```python
from build123d import *

# Parameters (mm, degrees)
SKETCH_31_W              = 54.5
SKETCH_31_H              = 38
EXTRUDE_11_DEPTH         = 4
SKETCH_32_W              = 4
SKETCH_32_H              = 38
EXTRUDE_12_DEPTH         = 28.5
SKETCH_33_W              = 16
SKETCH_33_H              = 38
EXTRUDE_13_DEPTH         = 4
SKETCH_34_W              = 15
SKETCH_34_H              = 4
EXTRUDE_14_DEPTH         = 28.5
HOLE_WIZARD_M2_5_1_D     = 2.9
HOLE_WIZARD_M2_5_1_DEPTH = 10
HOLE_WIZARD_M2_5_1_TIP   = 0.871247898
HOLE_WIZARD_M2_5_2_D     = 2.9
HOLE_WIZARD_M2_5_2_DEPTH = 10
HOLE_WIZARD_M2_5_2_TIP   = 0.871247898
HOLE_WIZARD_M2_5_3_D     = 2.9
HOLE_WIZARD_M2_5_3_DEPTH = 10
HOLE_WIZARD_M2_5_3_TIP   = 0.871247898
HOLE_WIZARD_M4_1_D       = 4.5
HOLE_WIZARD_M4_1_DEPTH   = 10
HOLE_WIZARD_M4_1_TIP     = 1.351936393
SKETCH_46_W              = 43
SKETCH_46_H              = 32.5
CUT_EXTRUDE_4_DEPTH      = 4


with BuildPart() as part:
    # 스케치31 → 보스-돌출11 (new body)
    with BuildSketch(Plane(origin=(0, 0, 0), x_dir=(1, 0, 0), z_dir=(0, 1, 0))):
        Rectangle(SKETCH_31_W, SKETCH_31_H)
    extrude(amount=EXTRUDE_11_DEPTH)

    # 스케치32 → 보스-돌출12 (add)
    with BuildSketch(Plane.XZ):
        with Locations((25.25, 0)):
            Rectangle(SKETCH_32_W, SKETCH_32_H)
        with Locations((-25.25, 0)):
            Rectangle(SKETCH_32_W, SKETCH_32_H)
    extrude(amount=EXTRUDE_12_DEPTH)

    # 스케치33 → 보스-돌출13 (add)
    with BuildSketch(Plane.XZ.offset(28.5)):
        with Locations((-35.25, 0)):
            Rectangle(SKETCH_33_W, SKETCH_33_H)
        with Locations((35.25, 0)):
            Rectangle(SKETCH_33_W, SKETCH_33_H)
    extrude(amount=-EXTRUDE_13_DEPTH)

    # 스케치34 → 보스-돌출14 (add)
    with BuildSketch(Plane.XZ):
        with Locations((-15.75, 17)):
            Rectangle(SKETCH_34_W, SKETCH_34_H)
    extrude(amount=EXTRUDE_14_DEPTH)

    # M2.5 여유 구멍1
    with Locations(Plane(origin=(0, 4, 0), x_dir=(1, 0, 0), z_dir=(0, 1, 0))):
        with Locations((8, 8), (8, -4), (-16, -4), (-16, 8)):
            Hole(HOLE_WIZARD_M2_5_1_D / 2, depth=HOLE_WIZARD_M2_5_1_DEPTH)
            with Locations((0, 0, -(HOLE_WIZARD_M2_5_1_DEPTH + HOLE_WIZARD_M2_5_1_TIP / 2))):  # 118° drill point
                Cone(0, HOLE_WIZARD_M2_5_1_D / 2, HOLE_WIZARD_M2_5_1_TIP, mode=Mode.SUBTRACT)

    # M2.5 여유 구멍2
    with Locations(Plane(origin=(27.25, 0, 0), x_dir=(0, 0, -1), z_dir=(1, 0, 0))):
        with Locations((-4, -6.25)):
            Hole(HOLE_WIZARD_M2_5_2_D / 2, depth=HOLE_WIZARD_M2_5_2_DEPTH)
            with Locations((0, 0, -(HOLE_WIZARD_M2_5_2_DEPTH + HOLE_WIZARD_M2_5_2_TIP / 2))):  # 118° drill point
                Cone(0, HOLE_WIZARD_M2_5_2_D / 2, HOLE_WIZARD_M2_5_2_TIP, mode=Mode.SUBTRACT)

    # M2.5 여유 구멍3
    with Locations(Plane.ZY.offset(27.25)):
        with Locations((4, -6.25), (-8, -6.25)):
            Hole(HOLE_WIZARD_M2_5_3_D / 2, depth=HOLE_WIZARD_M2_5_3_DEPTH)
            with Locations((0, 0, -(HOLE_WIZARD_M2_5_3_DEPTH + HOLE_WIZARD_M2_5_3_TIP / 2))):  # 118° drill point
                Cone(0, HOLE_WIZARD_M2_5_3_D / 2, HOLE_WIZARD_M2_5_3_TIP, mode=Mode.SUBTRACT)

    # M4 여유 구멍1
    with Locations(Plane(origin=(0, -24.5, 0), x_dir=(1, 0, 0), z_dir=(0, 1, 0))):
        with Locations((36.25, 10), (36.25, -10), (-36.25, -10), (-36.25, 10)):
            Hole(HOLE_WIZARD_M4_1_D / 2, depth=HOLE_WIZARD_M4_1_DEPTH)
            with Locations((0, 0, -(HOLE_WIZARD_M4_1_DEPTH + HOLE_WIZARD_M4_1_TIP / 2))):  # 118° drill point
                Cone(0, HOLE_WIZARD_M4_1_D / 2, HOLE_WIZARD_M4_1_TIP, mode=Mode.SUBTRACT)

    # 스케치46 → 컷-돌출4 (cut)
    with BuildSketch(Plane.XY.offset(19)):
        with Locations((21.75, -12.25)):
            Rectangle(SKETCH_46_W, SKETCH_46_H)
    extrude(amount=-CUT_EXTRUDE_4_DEPTH, mode=Mode.SUBTRACT)


solid = part.part
```
Part model, mm, in its own coordinate system. A direction names the side the tool comes from. Give positions to 0.01 mm unless a question says otherwise; leave off trailing zeros. Write each loop counter-clockwise with the first axis right and the second up, starting at its lowest first coordinate (ties: lowest second). Pieces come first, ordered by that corner, then holes. Notation, with made-up numbers: M 21,11 L 53,11 A16 ccw 53,34 Z; hole C 74,2.25 d1. An arc over 180 degrees is marked long. Use CSV: the item, a comma, the result in double quotes.
Item 1: Pull direction Z, two halves, no side cores. Call faces 1 (the face through (35.04, -26.528, 8.103)), 2 (the face through (23.25, -14, -2)), 3 (the face through (25, -10, 15)): +Z half, -Z half, draft (parallel to the pull), parting line (faces both ways), or undercut.
Taken from the geometry:
face 1,"undercut"
face 2,"draft"
face 3,"+Z half"
Item 2: Drill centre lines: probe 1 along X at (y, z) = (2.2, -8); probe 2 along Z at (x, y) = (-16, 1); probe 3 along X at (y, z) = (-26, 10). Where is each one in solid material? Low to high.
Taken from the geometry:
probe 1,"x = -27.25 to -17.45, -14.55 to 6.55, 9.45 to 27.25"
probe 2,"z = -19 to -9.45, -6.55 to 2.55, 5.45 to 19"
probe 3,"x = -43.25 to -38.5, -34 to -23.25, 23.25 to 34, 38.5 to 43.25"
Item 3: Slice it at D-D on y = -4. Write the cut outline in (x, z), plus the area to 3 significant figures.
Taken from the geometry:
outline,"M -27.25,-19 L -23.25,-19 L -23.25,15 L -8.25,15 L -8.25,19 L -27.25,19 Z; M 23.25,-19 L 27.25,-19 L 27.25,15 L 23.25,15 Z"
area,"348 mm²"
Item 4: Which spindle directions (+Z, -Z, +X, -X, +Y, -Y) get a long thin tool onto all of the face, cutting with end or side? Do faces 4 (the face through (-25.22, -6.19, -6.55)), 5 (the face through (-8.25, -14, 17)), 6 (the face through (27.25, -10, -2)), 7 (the face through (-23.25, -14, -2)). Say none if no direction does.
Taken from the geometry:
face 4,"-X"
face 5,"+Z, -Z, +X, -Y"
face 6,"+Z, -Z, +X, +Y"
face 7,"-Z, -Y"
Item 5: Slice it at B-B on x = -16. Write the cut outline in (y, z), plus the area to 3 significant figures.
Taken from the geometry:
outline,"M -28.5,15 L 0,15 L 0,5.45 L 4,5.45 L 4,19 L -28.5,19 Z; M 0,-19 L 4,-19 L 4,-9.45 L 0,-9.45 Z; M 0,-6.55 L 4,-6.55 L 4,2.55 L 0,2.55 Z"
area,"243 mm²"
Item 6: Pin check, flat tips, straight feed: P1, Ø3.5, axis at y = -6.25, z = -8, coming from the +X side; P2, Ø1.7, axis at y = -6.25, z = 4, coming from the -X side; P3, Ø10, axis at x = 22, y = -19.5, coming from the +Z side; P4, Ø1.5, axis at y = -3, z = 13, coming from the -X side. Stop position of each tip, or through.
Taken from the geometry:
P1,"stops at x = 27.25"
P2,"passes through"
P3,"stops at z = 15"
P4,"stops at x = -27.25"
Item 7: Slice it at C-C on z = 10. Write the cut outline in (x, y).
Taken from the geometry:
outline,"M -43.25,-28.5 L -38.5,-28.5 L -38.5,-24.5 L -43.25,-24.5 Z; M -34,-28.5 L -23.25,-28.5 L -23.25,0 L 23.25,0 L 23.25,-28.5 L 34,-28.5 L 34,-24.5 L 27.25,-24.5 L 27.25,4 L -27.25,4 L -27.25,-24.5 L -34,-24.5 Z; M 38.5,-28.5 L 43.25,-28.5 L 43.25,-24.5 L 38.5,-24.5 Z"
Item 8: Slice it at A-A on y = -25.5. Write the cut outline in (x, z), plus the area to 3 significant figures.
Taken from the geometry:
outline,"M -43.25,-19 L -23.25,-19 L -23.25,15 L -8.25,15 L -8.25,19 L -43.25,19 Z; M 23.25,-19 L 43.25,-19 L 43.25,15 L 23.25,15 Z; hole C -36.25,-10 d4.5; hole C -36.25,10 d4.5; hole C 36.25,-10 d4.5; hole C 36.25,10 d4.5"
area,"1,440 mm²"
